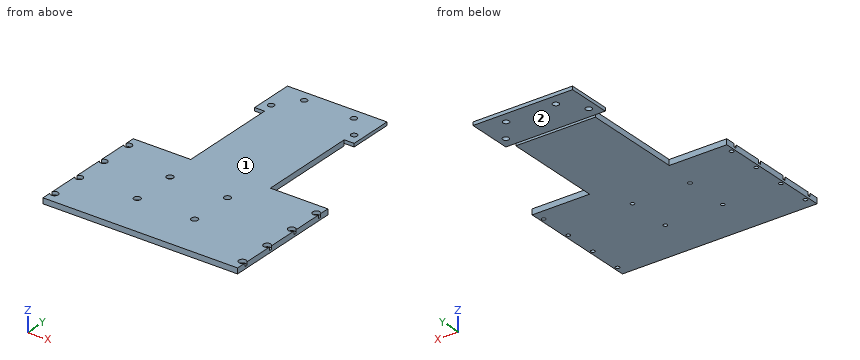
from build123d import *

# Parameters (mm, degrees)
EXTRUDE_1_DEPTH     = 3
SKETCH_2_W          = 72
SKETCH_2_H          = 200
EXTRUDE_2_DEPTH     = 2
SKETCH_4_R          = 2.75
CUT_EXTRUDE_1_DEPTH = 4
SKETCH_7_W          = 52
SKETCH_7_H          = 110
EXTRUDE_3_DEPTH     = 5
SKETCH_8_R          = 1.75
CUT_EXTRUDE_2_DEPTH = 6
SKETCH_9_R          = 3.25
CUT_EXTRUDE_3_DEPTH = 3
SKETCH_10_R         = 1.75
CUT_EXTRUDE_4_DEPTH = 6
SKETCH_11_R         = 3
CUT_EXTRUDE_5_DEPTH = 3


with BuildPart() as part:
    # ｽｹｯﾁ1 → ﾎﾞｽ - 押し出し1 (new body)
    with BuildSketch(Plane.XY):
        Polygon((-45, -20), (-36, -20), (-36, -220), (36, -220), (36, -20), (45, -20), (45, 20), (-45, 20), align=None)
    extrude_1 = extrude(amount=EXTRUDE_1_DEPTH)

    # ｽｹｯﾁ2 → ﾎﾞｽ - 押し出し2 (add)
    with BuildSketch(Plane(origin=(0, 0, 0), x_dir=(-1, 0, 0), z_dir=(0, 0, -1))):
        with Locations((0, -120)):
            Rectangle(SKETCH_2_W, SKETCH_2_H)
    extrude(amount=EXTRUDE_2_DEPTH)

    # ｽｹｯﾁ4 → ｶｯﾄ - 押し出し1 (cut, through all)
    with BuildSketch(Plane(origin=(0, 0, 0), x_dir=(-1, 0, 0), z_dir=(0, 0, -1))):
        with Locations((-22.5, 10)):
            Circle(SKETCH_4_R)
        with Locations((22.5, 10)):
            Circle(SKETCH_4_R)
        with Locations((37.5, -10)):
            Circle(SKETCH_4_R)
        with Locations((-37.5, -10)):
            Circle(SKETCH_4_R)
    cut_extrude_1 = extrude(amount=-CUT_EXTRUDE_1_DEPTH, mode=Mode.SUBTRACT)

    # ｽｹｯﾁ7 → ﾎﾞｽ - 押し出し3 (add)
    with BuildSketch(Plane.XY.offset(3)):
        with Locations((62, -165)):
            Rectangle(SKETCH_7_W, SKETCH_7_H)
    extrude_3 = extrude(amount=-EXTRUDE_3_DEPTH)

    # ｽｹｯﾁ8 → ｶｯﾄ - 押し出し2 (cut, through all)
    with BuildSketch(Plane.XY.offset(3)):
        with Locations((85, -180)):
            Circle(SKETCH_8_R)
        with Locations((85, -210)):
            Circle(SKETCH_8_R)
        with Locations((85, -150)):
            Circle(SKETCH_8_R)
        with Locations((85, -120)):
            Circle(SKETCH_8_R)
    cut_extrude_2 = extrude(amount=-CUT_EXTRUDE_2_DEPTH, mode=Mode.SUBTRACT)

    # ｽｹｯﾁ9 → ｶｯﾄ - 押し出し3 (cut)
    with BuildSketch(Plane.XY.offset(3)):
        with Locations((85, -180)):
            Circle(SKETCH_9_R)
        with Locations((85, -210)):
            Circle(SKETCH_9_R)
        with Locations((85, -150)):
            Circle(SKETCH_9_R)
        with Locations((85, -120)):
            Circle(SKETCH_9_R)
    cut_extrude_3 = extrude(amount=-CUT_EXTRUDE_3_DEPTH, mode=Mode.SUBTRACT)

    # ﾐﾗｰ1: ﾎﾞｽ - 押し出し1, ｶｯﾄ - 押し出し1, ﾎﾞｽ - 押し出し3, ｶｯﾄ - 押し出し2, ｶｯﾄ - 押し出し3 across plane
    add(extrude_1.mirror(Plane(origin=(0, 0, 0), x_dir=(0, 0, 1), z_dir=(1, 0, 0))))
    add(cut_extrude_1.mirror(Plane(origin=(0, 0, 0), x_dir=(0, 0, 1), z_dir=(1, 0, 0))), mode=Mode.SUBTRACT)
    add(extrude_3.mirror(Plane(origin=(0, 0, 0), x_dir=(0, 0, 1), z_dir=(1, 0, 0))))
    add(cut_extrude_2.mirror(Plane(origin=(0, 0, 0), x_dir=(0, 0, 1), z_dir=(1, 0, 0))), mode=Mode.SUBTRACT)
    add(cut_extrude_3.mirror(Plane(origin=(0, 0, 0), x_dir=(0, 0, 1), z_dir=(1, 0, 0))), mode=Mode.SUBTRACT)

    # ｽｹｯﾁ10 → ｶｯﾄ - 押し出し4 (cut, through all)
    with BuildSketch(Plane.XY.offset(3)):
        with Locations((19.5, -140)):
            Circle(SKETCH_10_R)
        with Locations((19.5, -180)):
            Circle(SKETCH_10_R)
        with Locations((-32.5, -180)):
            Circle(SKETCH_10_R)
        with Locations((-32.5, -140)):
            Circle(SKETCH_10_R)
    extrude(amount=-CUT_EXTRUDE_4_DEPTH, mode=Mode.SUBTRACT)

    # ｽｹｯﾁ11 → ｶｯﾄ - 押し出し5 (cut)
    with BuildSketch(Plane.XY.offset(3)):
        with Locations((-32.5, -140)):
            Circle(SKETCH_11_R)
        with Locations((19.5, -140)):
            Circle(SKETCH_11_R)
        with Locations((19.5, -180)):
            Circle(SKETCH_11_R)
        with Locations((-32.5, -180)):
            Circle(SKETCH_11_R)
    extrude(amount=-CUT_EXTRUDE_5_DEPTH, mode=Mode.SUBTRACT)


solid = part.part
Could you check a few things on this model? Use its own coordinates, in mm. Face numbers are marked on the shaded views. A direction names the side the tool comes from. Coordinates: 2 decimals unless noted, no trailing zeros. Order: outer loops, then holes, each group sorted by start corner. A loop starts at its lowest first (then second) coordinate and runs counter-clockwise, first axis right, second up. Notation, with made-up numbers: (26.5, 41.25) -> (59.5, 41.25) arc R32 cw to (59.5, 78.25) -> close; hole circle Ø7 at (-39, 45.5). An arc over 180 degrees is marked (long way). One line per question, with ' | ' between items.
Q1. I'm going to push flat-ended pins straight in: P1, Ø1.9, axis at x = -85.5, y = -178.5, coming from the +Z side; P2, Ø2, axis at y = -36, z = 2, coming from the +X side; P3, Ø3, axis at x = 85, y = -210, coming from the +Z side; P4, Ø6.5, axis at x = -37.5, y = -10, coming from the -Z side. Where does each tip first touch, or does it pass through?
Return value:
P1: z = 0 | P2: x = 36 | P3: through | P4: z = 0
Q2. If I drill on L1, parallel to Y at x = -85, z = -1.2; L2, parallel to X at y = -210, z = -1.25; L3, parallel to Y at x = -32.5, z = -1.3, over which ranges is the centre line in solid material (lowest first)?
Return value:
L1: -220 to -211.75, -208.25 to -181.75, -178.25 to -151.75, -148.25 to -121.75, -118.25 to -110 | L2: -88 to -86.75, -83.25 to 83.25, 86.75 to 88 | L3: -220 to -181.75, -178.25 to -141.75, -138.25 to -20
Q3. Imagine slicing it at A-A on y = -10. Please give me the cut outline in (x, z), and give its area (3 significant figures).
Return value:
outline: (-45, 0) -> (-40.25, 0) -> (-40.25, 3) -> (-45, 3) -> close; (-34.75, 0) -> (34.75, 0) -> (34.75, 3) -> (-34.75, 3) -> close; (40.25, 0) -> (45, 0) -> (45, 3) -> (40.25, 3) -> close | area: 237 mm²
Q4. On a 3-axis mill with a long thin cutter (end or side, diameter ignored), from which of +Z, -Z, +X, -X, +Y, -Y can I reach the whole of each face in a straight line? I mean the marked faces 1 and 2. Say none if no direction works.
Return value:
face 1: +Z, +X, -X, +Y, -Y | face 2: -Z, +X, -X, +Y
Q5. Imagine slicing it at B-B on x = -22.5. Please give me the cut outline in (y, z), and give its area (3 significant figures).
Return value:
outline: (-220, -2) -> (-20, -2) -> (-20, 0) -> (7.25, 0) -> (7.25, 3) -> (-220, 3) -> close; (12.75, 0) -> (20, 0) -> (20, 3) -> (12.75, 3) -> close | area: 1,100 mm²
Q6. Imagine slicing it at C-C on z = 1. State how many separate pieces and enclosed holes the cut face has, and give its area (3 significant figures).
Return value:
separate pieces: 1 | enclosed holes: 8 | area: 29,000 mm²
Q7. Imagine slicing it at D-D on x = 31.5. Please give me the cut outline in (y, z), and give its area (3 significant figures).
Return value:
outline: (-220, -2) -> (-20, -2) -> (-20, 0) -> (20, 0) -> (20, 3) -> (-220, 3) -> close | area: 1,120 mm²
